Design review of the part built by this model. Coordinates are the model's own, in mm. Face numbers are marked on the shaded views. A direction names the side the tool comes from. Coordinates: 2 decimals unless noted, no trailing zeros. Write each loop counter-clockwise with the first axis right and the second up, starting at its lowest first coordinate (ties: lowest second). Pieces come first, ordered by that corner, then holes. Notation, with made-up numbers: (-10.5, -15) - (-2.5, -15) arc R20 cw to (-2.5, 9) - close; hole circle Ø11 at (41.25, -38.75). An arc over 180 degrees is marked (long way). Use a Markdown table: item, result.
from build123d import *

# Parameters (mm, degrees)
SKETCH1_R           = 0.75
BOSS_EXTRUDE1_DEPTH = 15
CUT_EXTRUDE1_DEPTH  = 5


with BuildPart() as part:
    # Sketch1 → Boss-Extrude1 (new body)
    with BuildSketch(Plane(origin=(0, 0, 0), x_dir=(1, 0, 0), z_dir=(0, 1, 0))):
        with Locations(Location((0, 0, 0), (0, 0, 270))):
            Circle(SKETCH1_R)
    extrude(amount=BOSS_EXTRUDE1_DEPTH)

    # Sketch2 → Cut-Extrude1 (cut)
    with BuildSketch(Plane.XZ):
        with BuildLine():
            Line((-0.3, 0.687386354), (-0.3, -0.687386354))
            ThreePointArc((-0.3, -0.687386354), (-0.75, 0), (-0.3, 0.687386354))
        make_face()
        with BuildLine():
            Line((0.3, 0.687386354), (0.3, -0.687386354))
            ThreePointArc((0.3, -0.687386354), (0.75, 0), (0.3, 0.687386354))
        make_face()
    extrude(amount=-CUT_EXTRUDE1_DEPTH, mode=Mode.SUBTRACT)


solid = part.part
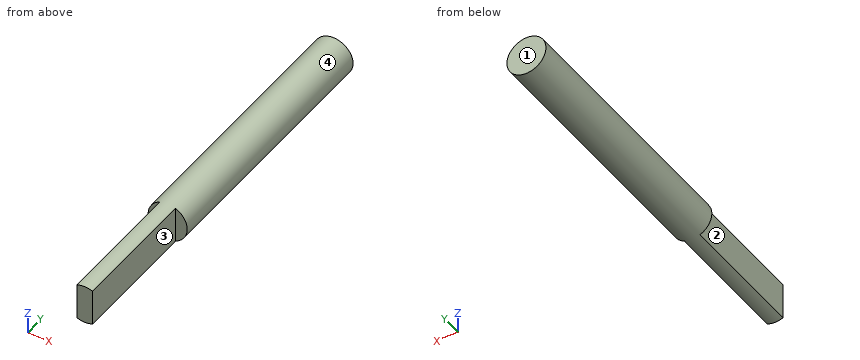
(1) Take a section at D-D on y = 3.75. Write out the cut boundary in (x, z).
Determined:
| item | result |
|---|---|
| outline | (-0.3, -0.69) arc R0.75 ccw to (0.3, -0.69) - (0.3, 0.69) arc R0.75 ccw to (-0.3, 0.69) - close |
(2) For L1, parallel to Y at x = -0.6, z = -0.3; L2, parallel to X at y = 1, z = -0.1; L3, parallel to Z at x = 0.05, y = 1.75, list the stretches that pass through material, from the lowest coordinate up. Write a range as from..to.
Determined:
| item | result |
|---|---|
| L1 | 5..15 |
| L2 | -0.3..0.3 |
| L3 | -0.75..0.75 |
(3) Machinability: for the marked faces 3 and 4, which of the approach directions +Z, -Z, +X, -X, +Y, -Y give a long, thin tool a straight path to every point of the face, cutting with its end or side? Answer none if there is none.
Determined:
| item | result |
|---|---|
| face 3 | +Z, -Z, +X, -Y |
| face 4 | +Y, -Y |
(4) For pin 1 (0.5 mm diameter, centred on x = -0.5, z = 0, fed in from -Y), flat-tipped, find the tip position at first contact; note if it passes through.
Determined:
| item | result |
|---|---|
| pin 1 | y = 0 |
(5) Take a section at A-A on z = 0. Write out the cut boundary in (x, y).
Determined:
| item | result |
|---|---|
| outline | (-0.75, 5) - (-0.3, 5) - (-0.3, 0) - (0.3, 0) - (0.3, 5) - (0.75, 5) - (0.75, 15) - (-0.75, 15) - close |
(6) Draft analysis for pull direction Y (two halves, no side actions). For the marked faces 1 and 2, state which applies: +Y half, -Y half, draft (parallel to the pull), parting line (faces both ways), or undercut.
Determined:
| item | result |
|---|---|
| face 1 | +Y half |
| face 2 | draft |
(7) Take a section at B-B on x = 0.45. Write out the cut boundary in (y, z).
Determined:
| item | result |
|---|---|
| outline | (5, -0.6) - (15, -0.6) - (15, 0.6) - (5, 0.6) - close |
(8) Take a section at C-C on y = 5.5. Write out the cut boundary in (x, z), and give its area (3 significant figures).
Determined:
| item | result |
|---|---|
| outline | circle Ø1.5 at (0, 0) |
| area | 1.77 mm2 |
